The listing builds one solid part. Answer for the finished solid, in the listing's coordinates (mm). A direction names the side the tool comes from. Coordinates: 2 decimals unless noted, no trailing zeros. Write each loop counter-clockwise with the first axis right and the second up, starting at its lowest first coordinate (ties: lowest second). Pieces come first, ordered by that corner, then holes.
```python
from build123d import *

# Parameters (mm, degrees)
F0_R           = 5.55625
F1_DEPTH       = 47.625
F0_R_2         = 6.5484375
F2_DEPTH       = 19.05
F4_DEPTH       = 28.575
F5_W           = 8.73125
F5_H           = 8.73125
F6_DEPTH       = 47.626
F7_R           = 4.365625
F8_DEPTH       = 9.525
F8_DEPTH_BACK  = 9.525
F10_DEPTH      = 9.525
F12_D          = 2.7051
F12_DEPTH      = 15.875
F12_TIP        = 0.8126940303
F14_DEPTH      = 3.175
F15_W          = 60.325
F15_H          = 50.8
F16_DEPTH      = 25.4
F16_DEPTH_BACK = 8.73225
F18_DEPTH      = 1.5875
F19_R          = 0.79375
F21_DEPTH      = 1.5875
F22_R          = 0.79375


# Not quite as in the source:
# - a pattern or mirror of a feature is missing from the dataset's text; its kind, count and spacing are read off the source's solid
# - a feature names something its author has since deleted; it is built from what else it names


with BuildPart() as f1:
    # F0 (on Right) → F1 (new body)
    with BuildSketch(Plane.YZ):
        with BuildLine():
            ThreePointArc((18.25625, -15.875), (16.6494169978, -11.0868310793), (12.4794785699, -8.2372543707))
            ThreePointArc((12.4794785699, -8.2372543707), (2.4565457231, -14.7842891497), (10.31875, -23.8125))
            ThreePointArc((10.31875, -23.8125), (15.9314100757, -21.4876600757), (18.25625, -15.875))
        make_face()
        with Locations((10.31875, -15.875)):
            Circle(F0_R, mode=Mode.SUBTRACT)
    extrude(amount=F1_DEPTH)



with BuildPart() as f1b:
    # F0 (on Right) → F1, piece 2 (new body)
    with BuildSketch(Plane.YZ):
        with BuildLine():
            ThreePointArc((-2.38125, -15.875), (-5.5305810793, -9.5443330022), (-12.4794785699, -8.2372543707))
            ThreePointArc((-12.4794785699, -8.2372543707), (-18.1809542769, -16.9657108503), (-10.31875, -23.8125))
            ThreePointArc((-10.31875, -23.8125), (-4.7060899243, -21.4876600757), (-2.38125, -15.875))
        make_face()
        with Locations((-10.31875, -15.875)):
            Circle(F0_R, mode=Mode.SUBTRACT)
    extrude(amount=F1_DEPTH)


with BuildPart() as f1_1:
    add(f1.part)

    add(f1b.part)  # F2 merges F1b
    # F0 (on Right) → F2 (join)
    with BuildSketch(Plane.YZ):
        with BuildLine():
            ThreePointArc((8.5506596809, -1.7666198185), (8.6859850881, -0.8879130653), (8.73125, 0))
            ThreePointArc((8.73125, 0), (-0.8879130653, 8.6859850881), (-8.5506596809, -1.7666198185))
            ThreePointArc((-8.5506596809, -1.7666198185), (0, -8.73125), (8.5506596809, -1.7666198185))
        make_face()
        Circle(F0_R_2, mode=Mode.SUBTRACT)
        with BuildLine():
            ThreePointArc((8.5506596809, -1.7666198185), (0, -8.73125), (-8.5506596809, -1.7666198185))
            ThreePointArc((-8.5506596809, -1.7666198185), (-9.2426468573, -5.7745223181), (-12.4794785699, -8.2372543707))
            ThreePointArc((-12.4794785699, -8.2372543707), (-5.5305810793, -9.5443330022), (-2.38125, -15.875))
            ThreePointArc((-2.38125, -15.875), (-4.7060899243, -21.4876600757), (-10.31875, -23.8125))
            Line((-10.31875, -23.8125), (10.31875, -23.8125))
            ThreePointArc((10.31875, -23.8125), (2.4565457231, -14.7842891497), (12.4794785699, -8.2372543707))
            ThreePointArc((12.4794785699, -8.2372543707), (9.2426468573, -5.7745223181), (8.5506596809, -1.7666198185))
        make_face()
    extrude(amount=F2_DEPTH)

    # F3 (on face) → F4 (join, through all)
    with BuildSketch(Plane.YZ.offset(47.625)):
        with BuildLine():
            ThreePointArc((5.9929049671, -9.2198537956), (0, -10.9963909515), (-5.9929049671, -9.2198537956))
            ThreePointArc((-5.9929049671, -9.2198537956), (-3.3423504559, -12.0890053287), (-2.38125, -15.875))
            ThreePointArc((-2.38125, -15.875), (-4.7060899243, -21.4876600757), (-10.31875, -23.8125))
            Line((-10.31875, -23.8125), (10.31875, -23.8125))
            ThreePointArc((10.31875, -23.8125), (2.7085880685, -18.1309569203), (5.9929049671, -9.2198537956))
        make_face()
    extrude(amount=-F4_DEPTH)

    # F5 (on face) → F6 (cut, through all)
    with BuildSketch(Plane(origin=(0, 0, 0), x_dir=(0, -1, 0), z_dir=(-1, 0, 0))):
        with Locations((0, -16.271875)):
            Rectangle(F5_W, F5_H)
    extrude(amount=-F6_DEPTH, mode=Mode.SUBTRACT)

    # F7 (on Front) → F8 (cut, two sides)
    with BuildSketch(Plane.XZ) as f8_sk:
        with Locations((0, -16.271875)):
            Circle(F7_R)
        with Locations((47.625, -16.271875)):
            Circle(F7_R)
    extrude(amount=-F8_DEPTH, mode=Mode.SUBTRACT)
    extrude(f8_sk.sketch, amount=F8_DEPTH_BACK, mode=Mode.SUBTRACT)

    # F9 (on face) → F10 (cut)
    with BuildSketch(Plane(origin=(0, 0, -11.90625), x_dir=(1, 0, 0), z_dir=(0, 0, -1))):
        with BuildLine():
            ThreePointArc((0, -4.3352987234), (2.7498472571, -2.8996680512), (3.8519455094, 0))
            ThreePointArc((3.8519455094, 0), (2.7498472571, 2.8996680512), (0, 4.3352987234))
            Line((0, 4.3352987234), (0, -4.3352987234))
        make_face()
        with BuildLine():
            Line((0, -4.3352987234), (0, 4.3352987234))
            ThreePointArc((0, 4.3352987234), (-4.8793044906, 0), (0, -4.3352987234))
        make_face()
    extrude(amount=-F10_DEPTH, mode=Mode.SUBTRACT)

    # F12
    with Locations(Plane(origin=(0, 0, 0), x_dir=(0, -1, 0), z_dir=(-1, 0, 0))):
        with Locations((7.14375, -7.9375), (-7.14375, -7.9375)):
            Hole(F12_D / 2, depth=F12_DEPTH)
            with Locations((0, 0, -(F12_DEPTH + F12_TIP / 2))):  # 118° drill point
                Cone(0, F12_D / 2, F12_TIP, mode=Mode.SUBTRACT)

    # F13 (on face) → F14 (join)
    with BuildSketch(Plane.YZ.offset(47.625)):
        with BuildLine():
            ThreePointArc((5.9929049671, -9.2198537956), (0, -10.9963909515), (-5.9929049671, -9.2198537956))
            ThreePointArc((-5.9929049671, -9.2198537956), (-17.9289119315, -13.6190430797), (-10.31875, -23.8125))
            Line((-10.31875, -23.8125), (10.31875, -23.8125))
            ThreePointArc((10.31875, -23.8125), (17.9289119315, -13.6190430797), (5.9929049671, -9.2198537956))
        make_face()
        with BuildLine():
            ThreePointArc((-7.4568436751, -20.6375), (-15.8369831688, -15.2261419591), (-6.4301850333, -11.90625))
            Line((-6.4301850333, -11.90625), (-4.365625, -11.90625))
            Line((-4.365625, -11.90625), (4.365625, -11.90625))
            Line((4.365625, -11.90625), (6.4301850333, -11.90625))
            ThreePointArc((6.4301850333, -11.90625), (12.4711991825, -10.7526102668), (15.875, -15.875))
            ThreePointArc((15.875, -15.875), (13.054663654, -20.7109787572), (7.4568436751, -20.6375))
            Line((7.4568436751, -20.6375), (4.365625, -20.6375))
            Line((4.365625, -20.6375), (-4.365625, -20.6375))
            Line((-4.365625, -20.6375), (-7.4568436751, -20.6375))
        make_face(mode=Mode.SUBTRACT)
        with BuildLine():
            Line((-4.365625, -11.90625), (-6.4301850333, -11.90625))
            ThreePointArc((-6.4301850333, -11.90625), (-15.8369831688, -15.2261419591), (-7.4568436751, -20.6375))
            Line((-7.4568436751, -20.6375), (-4.365625, -20.6375))
            Line((-4.365625, -20.6375), (4.365625, -20.6375))
            Line((4.365625, -20.6375), (7.4568436751, -20.6375))
            ThreePointArc((7.4568436751, -20.6375), (13.054663654, -20.7109787572), (15.875, -15.875))
            ThreePointArc((15.875, -15.875), (12.4711991825, -10.7526102668), (6.4301850333, -11.90625))
            Line((6.4301850333, -11.90625), (4.365625, -11.90625))
            Line((4.365625, -11.90625), (-4.365625, -11.90625))
        make_face()
    extrude(amount=F14_DEPTH)

    # F15 (on Top) → F16 (cut, two sides)
    with BuildSketch(Plane.XY) as f16_sk:
        with Locations((17.4625, 0)):
            Rectangle(F15_W, F15_H)
    extrude(amount=-F16_DEPTH, mode=Mode.SUBTRACT)
    extrude(f16_sk.sketch, amount=F16_DEPTH_BACK, mode=Mode.SUBTRACT)

    # F17 (on face) → F18 (join)
    with BuildSketch(Plane.YZ.offset(47.625)):
        with BuildLine():
            ThreePointArc((-7.4568436751, -20.6375), (-5.4827712428, -18.610913654), (-4.7625, -15.875))
            ThreePointArc((-4.7625, -15.875), (-5.1963602668, -13.7225508175), (-6.4301850333, -11.90625))
            ThreePointArc((-6.4301850333, -11.90625), (-15.8369831688, -15.2261419591), (-7.4568436751, -20.6375))
        make_face()
    f18 = extrude(amount=-F18_DEPTH)

    # F18_copies: F18 across plane
    add(f18.mirror(Plane.ZX))

    # F19
    f19_edges = [f1_1.edges().sort_by_distance(p)[0] for p in [
        (46.0375, 13.180656, -11.1125),
        (46.0375, -13.180656, -11.1125),
    ]]
    fillet(f19_edges, radius=F19_R)

    # F20 (on face) → F21 (cut)
    with BuildSketch(Plane(origin=(46.0375, 0, 0), x_dir=(0, -1, 0), z_dir=(-1, 0, 0))):
        with BuildLine():
            Line((6.7689920857, -12.7), (-12.7, -12.7))
            Line((-12.7, -12.7), (-12.7, -19.05))
            Line((-12.7, -19.05), (6.7689920857, -19.05))
            ThreePointArc((6.7689920857, -19.05), (5.55625, -15.875), (6.7689920857, -12.7))
        make_face()
        with BuildLine():
            Line((12.7, -12.7), (6.7689920857, -12.7))
            ThreePointArc((6.7689920857, -12.7), (5.55625, -15.875), (6.7689920857, -19.05))
            Line((6.7689920857, -19.05), (12.7, -19.05))
            Line((12.7, -19.05), (12.7, -12.7))
        make_face()
    extrude(amount=-F21_DEPTH, mode=Mode.SUBTRACT)

    # F22
    f22_edges = [f1_1.edges().sort_by_distance(p)[0] for p in [
        (50.8, 17.928912, -13.619043),
        (50.8, 0, -10.996391),
        (50.8, -17.928912, -13.619043),
        (50.8, 0, -23.8125),
    ]]
    fillet(f22_edges, radius=F22_R)


solid = f1_1.part
```
(1) Section A-A, the plane x = 48.95 is taken. Write down the section's boundary in (y, z) (1 decimal).
(2) Each of these flat-tipped pins is pushed along its axis until it touches: pin 1 (2 mm diameter, centred on x = 46.5, z = -12.5, fed in from +Y); pin 2 (1 mm diameter, centred on x = 49.5, z = -20, fed in from -Y); pin 3 (2 mm diameter, centred on x = 48, y = 5, fed in from +Z). Where does it stop, or does it pass through?
(3) Find the intervals of material crossed by probe 1 along X at (y, z) = (16, -16) (3 decimals); probe 2 along Y at (x, z) = (47.35, -11.5); probe 3 along Y at (x, z) = (46.75, -15.5), in increasing order.
(4) For a pull along Z with two mould halves and no side action, classify faces 1 (the flat face through (47, -9, -12.7)), 2 (the cylindrical face through (48.799, 17.985, -13.818)), 3 (the flat face through (46.038, -13, -16)) as pulls with the +Z half, pulls with the -Z half, needs draft (parallel to the pull), parting line crosses it, or undercut.
(5) Which of the six approach directions +Z, -Z, +X, -X, +Y, -Y give full straight-line access (tool end or side, diameter ignored) to faces 4 (the flat face through (47, -12.7, -16)), 5 (the flat face through (49, 0, -23.812))?
Solution:
1. outline: (-10.3, -23.8) - (10.3, -23.8) arc R7.9 ccw (long way) to (6, -9.2) arc R11 cw to (-6, -9.2) arc R7.9 ccw (long way) to start
2. pin 1: stops at y = 15.32
2. pin 2: stops at y = -17.38
2. pin 3: stops at z = -9.22
3. probe 1: x = 47.625 to 50.8
3. probe 2: y = -13.74 to -6.89, 6.89 to 13.74
3. probe 3: y = -15.86 to -12.7, 12.7 to 15.86
4. face 1: undercut
4. face 2: parting line crosses it
4. face 3: needs draft
5. face 4: -X
5. face 5: -Z, +X, -X, +Y, -Y
